Check sheet for the drawn part. Datum: minimum x, y, z corner. Units: mm. Give positions to 0.01 mm unless a question says otherwise; leave off trailing zeros. Order: outer loops, then holes, each group sorted by start corner. A loop starts at its lowest first (then second) coordinate and runs counter-clockwise, first axis right, second up. Notation, with made-up numbers: (56, 16.25) -> (96, 16.25) arc R17 ccw to (96, 30.25) -> close; hole circle Ø2 at (74.5, -2). An arc over 180 degrees is marked (long way). One line per question, with ' | ' between items. Start each with the question number.
Q1. Section check D-D on z = 11.65. Record the cut outline in (x, y) (1 decimal).
Q2. Section check A-A on x = 17.9. Record the cut outline in (y, z).
Q3. Material ranges on probe 1 along X at (y, z) = (1.7, 25); probe 2 along Z at (x, y) = (29, 0.75); probe 3 along X at (y, z) = (0.65, 11.65) (1 decimal), recorded low to high. Write a range as [from, to].
Q4. Section check C-C on z = 30.4. Record the cut outline in (x, y).
Q5. Go/stop test with a flat-tipped pin: pin 1 (1 mm diameter, centred on y = 1.5, z = 28, fed in from +X). Record where the tip stops, or that it passes through.
Q6. Section check B-B on y = 1.25. Give the number of separate pieces and of enclosed holes in the cut face, plus the area to 3 significant figures.
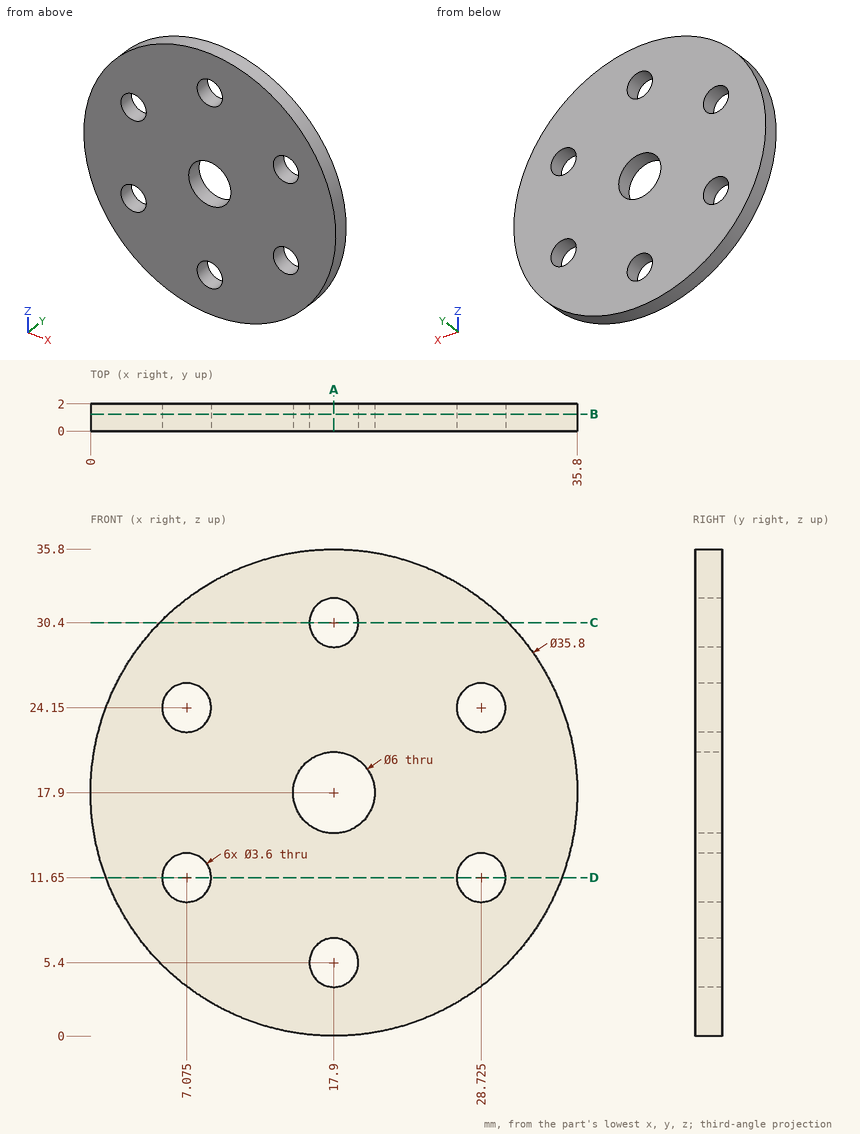
Filled in:
1) outline: (1.1, 0) -> (5.3, 0) -> (5.3, 2) -> (1.1, 2) -> close; (8.9, 0) -> (26.9, 0) -> (26.9, 2) -> (8.9, 2) -> close; (30.5, 0) -> (34.7, 0) -> (34.7, 2) -> (30.5, 2) -> close
2) outline: (0, 0) -> (2, 0) -> (2, 3.6) -> (0, 3.6) -> close; (0, 7.2) -> (2, 7.2) -> (2, 14.9) -> (0, 14.9) -> close; (0, 20.9) -> (2, 20.9) -> (2, 28.6) -> (0, 28.6) -> close; (0, 32.2) -> (2, 32.2) -> (2, 35.8) -> (0, 35.8) -> close
3) probe 1: [1.47, 5.49], [8.66, 27.14], [30.31, 34.33] | probe 2: [3.86, 9.87], [13.43, 22.37], [25.93, 31.94] | probe 3: [1.1, 5.3], [8.9, 26.9], [30.5, 34.7]
4) outline: (5.09, 0) -> (16.1, 0) -> (16.1, 2) -> (5.09, 2) -> close; (19.7, 0) -> (30.71, 0) -> (30.71, 2) -> (19.7, 2) -> close
5) pin 1: x = 33.01
6) separate pieces: 1 | enclosed holes: 7 | area: 917 mm²
